```python
from build123d import *

# Parameters (mm, degrees)
SKETCH1_R               = 1.6
BOSS_EXTRUDE1_DEPTH     = 10
CUT_EXTRUDE1_START      = -7
CUT_EXTRUDE1_DEPTH      = 4
FILLET1_R               = 5
CUT_EXTRUDE2_START      = 49.5
CUT_EXTRUDE2_OUTLINE_W  = 4
CUT_EXTRUDE2_OUTLINE_H  = 10
CUT_EXTRUDE2_DEPTH      = 10.5
CUT_EXTRUDE3_DEPTH      = 62.64414003
CUT_EXTRUDE3_DEPTH_BACK = 62.64414003
SKETCH5_R               = 1.6
CHAMFER1_SIZE           = 0.5


# Read off the part's stored shape, not the designer's step: Cut-Extrude2
with BuildPart() as part:
    # Sketch1 → Boss-Extrude1 (new body)
    with BuildSketch(Plane.XY):
        with BuildLine():
            Line((0, 5), (60, 5))
            Line((60, 5), (60, -5))
            Line((60, -5), (0, -5))
            ThreePointArc((0, -5), (-5, 0), (0, 5))
        make_face()
        Circle(SKETCH1_R, mode=Mode.SUBTRACT)
    extrude(amount=BOSS_EXTRUDE1_DEPTH)

    # Sketch2 → Cut-Extrude1 (cut)
    with BuildSketch(Plane.XY.offset(10).offset(CUT_EXTRUDE1_START)):
        with BuildLine():
            Line((5.5, 5), (5.5, -5))
            Line((5.5, -5), (0, -5))
            ThreePointArc((0, -5), (-5, 0), (0, 5))
            Line((0, 5), (5.5, 5))
        make_face()
    extrude(amount=CUT_EXTRUDE1_DEPTH, mode=Mode.SUBTRACT)

    # Fillet1
    fillet1_edges = [part.edges().sort_by_distance(p)[0] for p in [
        (60, 0, 0),
        (60, 0, 10),
    ]]
    fillet(fillet1_edges, radius=FILLET1_R - 0.0001)  # a hair under: the kernel refuses the full size

    # Cut-Extrude2 outline → Cut-Extrude2 (cut)
    with BuildSketch(Plane.YZ.offset(CUT_EXTRUDE2_START)):
        with Locations((0, 5)):
            Rectangle(CUT_EXTRUDE2_OUTLINE_W, CUT_EXTRUDE2_OUTLINE_H)
    extrude(amount=CUT_EXTRUDE2_DEPTH, mode=Mode.SUBTRACT)

    # Sketch5 → Cut-Extrude3 (cut, two sides: drawn at the far end of the back side and taken through both)
    with BuildSketch(Plane(origin=(0, 5, 0), x_dir=(1, 0, 0), z_dir=(0, 1, 0)).offset(-CUT_EXTRUDE3_DEPTH_BACK)):
        with Locations(Location((55, -5, 0), (0, 0, 270))):
            Circle(SKETCH5_R)
    extrude(amount=CUT_EXTRUDE3_DEPTH + CUT_EXTRUDE3_DEPTH_BACK, mode=Mode.SUBTRACT)

    # Chamfer1
    chamfer1_edges = [part.edges().sort_by_distance(p)[0] for p in [
        (-1.6, 0, 0),
        (-1.6, 0, 10),
        (-1.6, 0, 3),
        (2.75, 5, 3),
        (5.5, 5, 5),
        (2.75, -5, 3),
        (5.5, -5, 5),
        (-5, 0, 3),
        (-1.6, 0, 7),
        (2.75, 5, 7),
        (-5, 0, 7),
        (2.75, -5, 7),
        (27.50005, 5, 10),
        (27.50005, 5, 0),
        (58.535563195, 5, 8.535563195),
        (58.535563195, 5, 1.464436805),
        (58.535563195, -5, 8.535563195),
        (58.535563195, -5, 1.464436805),
        (-5, 0, 10),
        (58.535563195, 2, 1.464436805),
        (58.535563195, -2, 1.464436805),
        (58.535563195, -2, 8.535563195),
        (27.50005, -5, 0),
        (52.25005, -2, 10),
        (49.5, 0, 10),
        (52.25005, -2, 0),
        (49.5, 0, 0),
        (58.535563195, 2, 8.535563195),
        (52.25005, 2, 0),
        (52.25005, 2, 10),
        (-5, 0, 0),
        (55, 2, 3.4),
        (55, 5, 3.4),
        (55, -2, 3.4),
        (55, -5, 3.4),
        (27.50005, -5, 10),
    ]]
    chamfer(chamfer1_edges, length=CHAMFER1_SIZE)


solid = part.part
```
Verification items for the finished model (mm, model axes). A direction names the side the tool comes from. Round coordinates to 2 decimals unless told otherwise and drop trailing zeros. Write each loop counter-clockwise with the first axis right and the second up, starting at its lowest first coordinate (ties: lowest second). Pieces come first, ordered by that corner, then holes.
1. Gauge pin test, flat ends, axial feed: P1, Ø3.5, axis at x = 55, z = 5, coming from the +Y side; P2, Ø4, axis at x = 0, y = 0, coming from the +Z side; P3, Ø1.2, axis at y = 0.5, z = 3, coming from the +X side. Record the tip position at first contact, or that the pin passes through.
2. Access from +Z, -Z, +X, -X, +Y, -Y to the whole of each face (thin tool, end or side, straight path). Record for faces 5 (the flat face through (29, 5, 5)), 6 (the flat face through (3, 0, 7)), 7 (the cylindrical face through (58, -4, 1)), 8 (the conical face through (58.314, -2.135, 8.242)), 9 (the flat face through (52, -2, 5)).
3. Section check A-A on y = 0. State how many separate pieces and enclosed holes the cut face has, plus the area to 3 significant figures.
4. Scan lines: L1, parallel to X at y = 3.7, z = 5; L2, parallel to Y at x = 0, z = 8.3; L3, parallel to Z at x = 55, y = 3.75. Record each from-to range of solid material in increasing order.
5. Draft check along Z on faces 1 (the flat face through (52, 2, 5)), 2 (the cylindrical face through (56.35, 3.49, 5.86)), 3 (the conical face through (58.314, 2.135, 8.242)), 4 (the conical face through (58.242, 2.135, 1.686)). Enter one of: +Z half, -Z half, draft (parallel to the pull), parting line (faces both ways), or undercut.
6. Section check B-B on x = 4. Enter the section's corners in (y, z), plus the area to 3 significant figures.
Answer:
1. P1: stops at y = 4.65
1. P2: stops at z = 9.9
1. P3: stops at x = 49.5
2. face 5: +Z, -Z, +X, -X, +Y
2. face 6: -X, +Y, -Y
2. face 7: -Z, +X, +Y, -Y
2. face 8: +Z, +X
2. face 9: +Z, -Z, +X
3. separate pieces: 3
3. enclosed holes: 0
3. area: 482 mm2
4. L1: x = 5.5 to 53.4, 56.6 to 60
4. L2: y = -5 to -1.6, 1.6 to 5
4. L3: z = 0 to 3.4, 6.6 to 10
5. face 1: draft
5. face 2: undercut
5. face 3: +Z half
5. face 4: -Z half
6. outline: (-5, 0.5) - (-4.5, 0) - (4.5, 0) - (5, 0.5) - (5, 2.5) - (4.5, 3) - (-4.5, 3) - (-5, 2.5) - close; (-5, 7.5) - (-4.5, 7) - (4.5, 7) - (5, 7.5) - (5, 9.5) - (4.5, 10) - (-4.5, 10) - (-5, 9.5) - close
6. area: 59.0 mm2
